from build123d import *

# Parameters (mm, degrees)
SKETCH_W      = 28
SKETCH_H      = 15
SKETCH_R      = 5.9
SKETCH_R_2    = 1.64
PAD_DEPTH     = 2
SKETCH001_R   = 3
SKETCH001_R_2 = 1.64
PAD001_DEPTH  = 1.6
FILLET_R      = 4


with BuildPart() as part:
    # Sketch → Pad (new body)
    with BuildSketch(Plane.XY):
        Rectangle(SKETCH_W, SKETCH_H)
        Circle(SKETCH_R, mode=Mode.SUBTRACT)
        with Locations((-11, 0)):
            Circle(SKETCH_R_2, mode=Mode.SUBTRACT)
        with Locations((11, 0)):
            Circle(SKETCH_R_2, mode=Mode.SUBTRACT)
    extrude(amount=PAD_DEPTH)

    # Sketch001 (on Face9 of Pad) → Pad001 (join)
    with BuildSketch(Plane.XY.offset(2)):
        with Locations((-11, 0)):
            Circle(SKETCH001_R)
        with Locations((-11, 0)):
            Circle(SKETCH001_R_2, mode=Mode.SUBTRACT)
        with Locations((11, 0)):
            Circle(SKETCH001_R)
        with Locations((11, 0)):
            Circle(SKETCH001_R_2, mode=Mode.SUBTRACT)
    extrude(amount=PAD001_DEPTH)

    # Fillet
    fillet_edges = [part.edges().sort_by_distance(p)[0] for p in [
        (14, -7.5, 1),
        (14, 7.5, 1),
        (-14, 7.5, 1),
        (-14, -7.5, 1),
    ]]
    fillet(fillet_edges, radius=FILLET_R)


solid = part.part
For this review, take the finished solid that the model builds, in its own axes (mm). A direction names the side the tool comes from. Coordinates: 2 decimals unless noted, no trailing zeros. Order: outer loops, then holes, each group sorted by start corner. A loop starts at its lowest first (then second) coordinate and runs counter-clockwise, first axis right, second up. Notation, with made-up numbers: (65.5, 34.25) - (87.5, 34.25) arc R24 cw to (87.5, 53.25) - close; hole circle Ø3 at (76, -26). An arc over 180 degrees is marked (long way). Answer as CSV lines item,"result". Start each with the question number.
1) Draft analysis for pull direction Y (two halves, no side actions). For faces 1 (the cylindrical face through (-12.64, 0.07, 1.77)), 2 (the flat face through (-14, 0, 1)), 3 (the cylindrical face through (12.859, 6.297, 1.014)), state which applies: +Y half, -Y half, draft (parallel to the pull), parting line (faces both ways), or undercut.
2) Machinability: for faces 4 (the cylindrical face through (-12.797, 6.359, 1.014)), 5 (the cylindrical face through (-13.4, -1.8, 2.8)), which of the approach directions +Z, -Z, +X, -X, +Y, -Y give a long, thin tool a straight path to every point of the face, cutting with its end or side? Answer none if there is none.
3) Insertion check: P1, Ø8, axis at x = 6.5, y = 6, coming from the -Z side. The pin has a flat end and moves straight along its axis. Give the tip position at first contact, or say it passes through.
4) To check wall thickness, follow line 1 along Y through (x, z) = (0, 1.65); line 2 along X through (y, z) = (1, 2.4); line 3 along Z through (x, y) = (-8.5, 7). State the ranges of each line that lie inside material, in increasing order. Write a range as [from, to].
5) Add section C-C (z = 2.85). State the section outline as (x, y) points.
6) Add section D-D (x = 11.5). State the section outline as (y, z) points, then the cut area to 3 significant figures.
7) Add section A-A (x = 0). State the section outline as (y, z) points, then the cut area to 3 significant figures.
8) Add section B-B (z = 0.6). State the section outline as (x, y) points.
Result:
1,face 1,"undercut"
1,face 2,"draft"
1,face 3,"+Y half"
2,face 4,"+Z, -Z, -X, +Y"
2,face 5,"+Z"
3,P1,"z = 0"
4,line 1,"[-7.5, -5.9], [5.9, 7.5]"
4,line 2,"[-13.83, -12.3], [-9.7, -8.17], [8.17, 9.7], [12.3, 13.83]"
4,line 3,"[0, 2]"
5,outline,"circle Ø6 at (-11, 0); circle Ø6 at (11, 0); hole circle Ø3.28 at (-11, 0); hole circle Ø3.28 at (11, 0)"
6,outline,"(-7.21, 0) - (-1.56, 0) - (-1.56, 3.6) - (-2.96, 3.6) - (-2.96, 2) - (-7.21, 2) - close; (1.56, 0) - (7.21, 0) - (7.21, 2) - (2.96, 2) - (2.96, 3.6) - (1.56, 3.6) - close"
6,area,"27.1 mm^2"
7,outline,"(-7.5, 0) - (-5.9, 0) - (-5.9, 2) - (-7.5, 2) - close; (5.9, 0) - (7.5, 0) - (7.5, 2) - (5.9, 2) - close"
7,area,"6.40 mm^2"
8,outline,"(-14, -3.5) arc R4 ccw to (-10, -7.5) - (10, -7.5) arc R4 ccw to (14, -3.5) - (14, 3.5) arc R4 ccw to (10, 7.5) - (-10, 7.5) arc R4 ccw to (-14, 3.5) - close; hole circle Ø3.28 at (-11, 0); hole circle Ø11.8 at (0, 0); hole circle Ø3.28 at (11, 0)"
